```python
from build123d import *

# Parameters (mm, degrees)
F0_R             = 46
F1_DEPTH         = 22.5
F2_T             = -8.5
F3_R             = 55.4976575172
F3_R_2           = 39
F4_DEPTH         = 0.3
F5_R             = 5
F6_DEPTH         = 6
F7_R             = 7.5
F7_R_2           = 5
F8_DEPTH         = 5
F9_SIZE2         = 5
F9_SIZE          = 5
F10_W            = 11.5703346615
F10_H            = 10
F11_DEPTH        = 22.501
F11_COPIES_COUNT = 4


# Not quite as in the source:
# - a pattern or mirror of a feature is missing from the dataset's text; its kind, count and spacing are read off the source's solid


with BuildPart() as f1:
    # F0 (on Front) → F1 (new body)
    with BuildSketch(Plane.XZ):
        Circle(F0_R)
    extrude(amount=F1_DEPTH)

    # F2
    f2_openings = [f1.faces().sort_by_distance(p)[0] for p in [
        (0, -22.5, 0),
    ]]
    offset(amount=F2_T, openings=f2_openings)

    # F3 (on Front) → F4 (cut)
    with BuildSketch(Plane.XZ):
        Circle(F3_R)
        Circle(F3_R_2, mode=Mode.SUBTRACT)
    extrude(amount=F4_DEPTH, mode=Mode.SUBTRACT)

    # F5 (on Front) → F6 (join)
    with BuildSketch(Plane.XZ):
        Circle(F5_R)
    extrude(amount=-F6_DEPTH)

    # F7 (on face) → F8 (join)
    with BuildSketch(Plane(origin=(0, 6, 0), x_dir=(-1, 0, 0), z_dir=(0, 1, 0))):
        Circle(F7_R)
        Circle(F7_R_2, mode=Mode.SUBTRACT)
        Circle(F7_R_2)
    extrude(amount=F8_DEPTH)

    # F9
    f9_edges = [f1.edges().sort_by_distance(p)[0] for p in [
        (-46, -0.3, 0),
        (-46, -22.5, 0),
    ]]
    chamfer(f9_edges, length=F9_SIZE, length2=F9_SIZE2)

    # F10 (on Front) → F11 (cut, through all)
    with BuildSketch(Plane.XZ):
        with Locations((46.7851673308, 0)):
            Rectangle(F10_W, F10_H)
    f11 = extrude(amount=F11_DEPTH, mode=Mode.SUBTRACT)

    # F11_copies: F11 ×4 about axis
    f11_copies_axis = Axis((0, 0, 0), (0, 1, 0))
    for i in range(1, F11_COPIES_COUNT):
        add(f11.rotate(f11_copies_axis, i * 360 / F11_COPIES_COUNT), mode=Mode.SUBTRACT)


solid = f1.part
```
Verification items for the finished model (mm, model axes). A direction names the side the tool comes from. Round coordinates to 2 decimals unless told otherwise and drop trailing zeros. Write each loop counter-clockwise with the first axis right and the second up, starting at its lowest first coordinate (ties: lowest second). Pieces come first, ordered by that corner, then holes.
1. Gauge pin test, flat ends, axial feed: P1, Ø2.5, axis at x = -43.5, y = -16, coming from the -Z side; P2, Ø4, axis at y = -15.5, z = -31.5, coming from the -X side; P3, Ø16.5, axis at x = -0.5, z = -2, coming from the -Y side. Record the tip position at first contact, or that the pin passes through.
2. Draft check along X on faces 6 (the flat face through (41, -11, 0)), 7 (the flat face through (0, -11, 41)), 8 (the flat face through (-41, -11, 0)), 9 (the flat face through (5, -11, 43)). Enter one of: +X half, -X half, draft (parallel to the pull), parting line (faces both ways), or undercut.
3. Section check A-A on y = -20. Enter the section's corners in (x, z).
4. Section check B-B on y = 1.5. Enter the section's corners in (x, z).
5. Access from +Z, -Z, +X, -X, +Y, -Y to the whole of each face (thin tool, end or side, straight path). Record for faces 1 (the flat face through (36.3, -0.3, -15)), 2 (the flat face through (-2, 6, -5)), 3 (the flat face through (-5, -11, 43)), 4 (the flat face through (-43, -11, 5)), 5 (the flat face through (0, -11, -41)).
6. Scan lines: L1, parallel to Z at x = 0, y = -16.75; L2, parallel to Y at x = 19.5, z = 27.5. Record each from-to range of solid material in increasing order.
Answer:
1. P1: stops at z = -18.19
1. P2: stops at x = -35.3
1. P3: stops at y = -8.5
2. face 6: +X half
2. face 7: undercut
2. face 8: -X half
2. face 9: undercut
3. outline: (-43.21, -5) arc R43.5 ccw to (-5, -43.21) - (-5, -41) - (5, -41) - (5, -43.21) arc R43.5 ccw to (43.21, -5) - (41, -5) - (41, 5) - (43.21, 5) arc R43.5 ccw to (5, 43.21) - (5, 41) - (-5, 41) - (-5, 43.21) arc R43.5 ccw to (-43.21, 5) - (-41, 5) - (-41, -5) - close; hole circle Ø75 at (0, 0)
4. outline: circle Ø10 at (0, 0)
5. face 1: +Y
5. face 2: none
5. face 3: +Z, +Y, -Y
5. face 4: -X, +Y, -Y
5. face 5: -Z, +Y, -Y
6. L1: z = -41 to -37.5, 37.5 to 41
6. L2: y = -8.5 to 0
